from build123d import *

# Parameters (mm, degrees)
SKETCH1_R           = 5
BOSS_EXTRUDE1_DEPTH = 103
SKETCH5_W           = 1
SKETCH5_H           = 4
SKETCH6_R           = 5
CUT_EXTRUDE1_DEPTH  = 20


with BuildPart() as part:
    # Sketch1 → Boss-Extrude1 (new body)
    with BuildSketch(Plane(origin=(0, 0, 0), x_dir=(1, 0, 0), z_dir=(0, 1, 0))):
        with Locations(Location((0, 0, 0), (0, 0, 270))):
            Circle(SKETCH1_R)
    extrude(amount=BOSS_EXTRUDE1_DEPTH)

    # Sketch4 → Ø4.0mm Dowel Hole1 (revolve, cut)
    with BuildSketch(Plane(origin=(0, 103, 0), x_dir=(0, 0, 1), z_dir=(1, 0, 0))):
        Polygon((0, 0), (0, 19.201721238), (2, 18), (2, 0.025), (2.025, 0), align=None)
    f_4_0mm_dowel_hole1 = revolve(axis=Axis((0, 109.35, 0), (0, -1, 0)), mode=Mode.SUBTRACT)

    # Mirror1: Ø4.0mm Dowel Hole1 across plane
    add(f_4_0mm_dowel_hole1.mirror(Plane.ZX.offset(51.5)), mode=Mode.SUBTRACT)

    # Sketch5 → Cut-Revolve2 (revolve, cut)
    with BuildSketch(Plane.XY):
        with Locations((-4.5, 101)):
            Rectangle(SKETCH5_W, SKETCH5_H)
        with Locations((-4.5, 2)):
            Rectangle(SKETCH5_W, SKETCH5_H)
    revolve(axis=Axis((0, 103, 0), (0, -1, 0)), mode=Mode.SUBTRACT)

    # Sketch6 → Cut-Extrude1 (cut)
    with BuildSketch(Plane(origin=(0, 99, 0), x_dir=(1, 0, 0), z_dir=(0, 1, 0))):
        with Locations(Location((0, 0, 0), (0, 0, 180))):
            Circle(SKETCH6_R)
    cut_extrude1 = extrude(amount=CUT_EXTRUDE1_DEPTH, mode=Mode.SUBTRACT)

    # Mirror3: Cut-Extrude1 across plane
    add(cut_extrude1.mirror(Plane.ZX.offset(51.5)), mode=Mode.SUBTRACT)


solid = part.part
Check sheet for the modelled part. Datum: model origin and axes. Units: mm. A direction names the side the tool comes from. Coordinates: 2 decimals unless noted, no trailing zeros. Write each loop counter-clockwise with the first axis right and the second up, starting at its lowest first coordinate (ties: lowest second). Pieces come first, ordered by that corner, then holes.
Item 1: Cross-section at A-A on y = 65. Record the boundary of the cut face in (x, z).
Numbers:
outline: circle Ø10 at (0, 0)
Item 2: Depth check by flat-ended pin: pin 1 Ø1.5 at (y, z) = (48, 1) entering from +X; pin 2 Ø1 at (y, z) = (61, -3.5) entering from -X; pin 3 Ø2 at (x, y) = (3, 58.5) entering from +Z. Enter the tip coordinate at first touch or a pass-through.
Numbers:
pin 1: stops at x = 4.99
pin 2: stops at x = -4
pin 3: stops at z = 4.58
Item 3: Access from +Z, -Z, +X, -X, +Y, -Y to the whole of each face (thin tool, end or side, straight path). Record for faces 4 (the face through (-2.2, 4, -0.1)), 5 (the face through (2, 92, 0)), 6 (the face through (2, 11, 0)).
Numbers:
face 4: +Z, -Z, +X, -X, -Y
face 5: +Y
face 6: -Y
Item 4: Mould release check, pull along X, two halves, no side actions. Record for faces 1 (the face through (0.34, 18.99, -0.08)), 2 (the face through (0.1, 99, 2.2)), 3 (the face through (1.5, 50.84, 4.77)): released by +X, released by -X, zero draft, split by the parting line, or undercut.
Numbers:
face 1: undercut
face 2: zero draft
face 3: split by the parting line
Item 5: Cross-section at B-B on x = -3. Record the boundary of the cut face in (y, z), then the cut area to 3 significant figures.
Numbers:
outline: (4, -4) - (99, -4) - (99, 4) - (4, 4) - close
area: 760 mm2
Item 6: Scan lines: probe 1 along X at (y, z) = (13.75, 0); probe 2 along X at (y, z) = (36, -1.25); probe 3 along X at (y, z) = (93.5, -3). Record each from-to range of solid material in increasing order.
Numbers:
probe 1: x = -5 to -2, 2 to 5
probe 2: x = -4.84 to 4.84
probe 3: x = -4 to 4
Item 7: Cross-section at C-C on x = 3.5. Record the boundary of the cut face in (y, z).
Numbers:
outline: (4, -3.57) - (99, -3.57) - (99, 3.57) - (4, 3.57) - close
